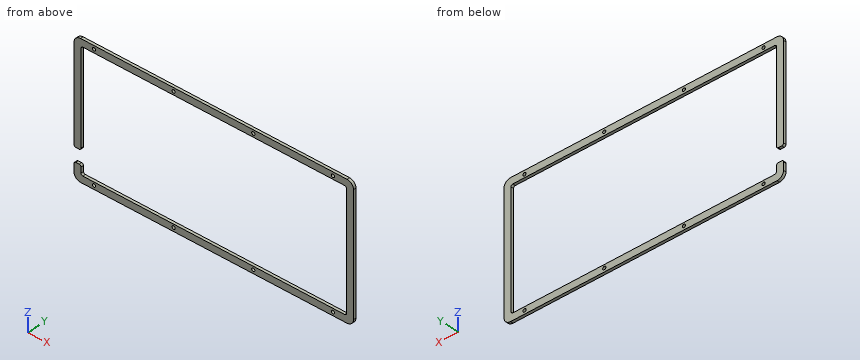
from build123d import *

# Parameters (mm, degrees)
SKETCH1_W           = 350
SKETCH1_H           = 200
BOSS_EXTRUDE1_DEPTH = 3
SKETCH2_OUTSIDE_W   = 432.624
SKETCH2_OUTSIDE_H   = 282.624
SKETCH2_OUTSIDE_R   = 1.7
CUT_EXTRUDE1_DEPTH  = 10


with BuildPart() as part:
    # Sketch1 → Boss-Extrude1 (new body)
    with BuildSketch(Plane(origin=(0, 0, 0), x_dir=(1, 0, 0), z_dir=(0, 1, 0))):
        with Locations((175, 100)):
            Rectangle(SKETCH1_W, SKETCH1_H)
    extrude(amount=BOSS_EXTRUDE1_DEPTH)

    # Sketch2 outside → Cut-Extrude1 (cut)
    with BuildSketch(Plane(origin=(0, 3, 0), x_dir=(1, 0, 0), z_dir=(0, 1, 0))):
        with Locations((175, 100)):
            Rectangle(SKETCH2_OUTSIDE_W, SKETCH2_OUTSIDE_H)
        with BuildLine():
            Line((334.453835379, 22.4974157), (46.754485379, 22.4974157))
            ThreePointArc((46.754485379, 22.4974157), (41.80473791, 24.547668232), (39.754485379, 29.4974157))
            Line((39.754485379, 29.4974157), (39.754485379, 132.1968757))
            ThreePointArc((39.754485379, 132.1968757), (40.340271816, 133.611089262), (41.754485379, 134.1968757))
            Line((41.754485379, 134.1968757), (45.254485379, 134.1968757))
            ThreePointArc((45.254485379, 134.1968757), (46.668698941, 133.611089262), (47.254485379, 132.1968757))
            Line((47.254485379, 132.1968757), (47.254485379, 31.9974157))
            ThreePointArc((47.254485379, 31.9974157), (47.840271816, 30.583202138), (49.254485379, 29.9974157))
            Line((49.254485379, 29.9974157), (331.953835379, 29.9974157))
            ThreePointArc((331.953835379, 29.9974157), (333.368048941, 30.583202138), (333.953835379, 31.9974157))
            Line((333.953835379, 31.9974157), (333.953835379, 157.1968757))
            ThreePointArc((333.953835379, 157.1968757), (333.368048941, 158.611089262), (331.953835379, 159.1968757))
            Line((331.953835379, 159.1968757), (49.254485379, 159.1968757))
            ThreePointArc((49.254485379, 159.1968757), (47.840271816, 158.611089262), (47.254485379, 157.1968757))
            Line((47.254485379, 157.1968757), (47.254485379, 151.1968757))
            ThreePointArc((47.254485379, 151.1968757), (46.668698941, 149.782662138), (45.254485379, 149.1968757))
            Line((45.254485379, 149.1968757), (41.754485379, 149.1968757))
            ThreePointArc((41.754485379, 149.1968757), (40.340271816, 149.782662138), (39.754485379, 151.1968757))
            Line((39.754485379, 151.1968757), (39.754485379, 159.6968757))
            ThreePointArc((39.754485379, 159.6968757), (41.80473791, 164.646623168), (46.754485379, 166.6968757))
            Line((46.754485379, 166.6968757), (334.453835379, 166.6968757))
            ThreePointArc((334.453835379, 166.6968757), (339.403582847, 164.646623168), (341.453835379, 159.6968757))
            Line((341.453835379, 159.6968757), (341.453835379, 29.4974157))
            ThreePointArc((341.453835379, 29.4974157), (339.403582847, 24.547668232), (334.453835379, 22.4974157))
        make_face(mode=Mode.SUBTRACT)
        with Locations((319.254485379, 26.4974157)):
            Circle(SKETCH2_OUTSIDE_R)
        with Locations((233.254485379, 26.2474157)):
            Circle(SKETCH2_OUTSIDE_R)
        with Locations((61.254485379, 26.2474157)):
            Circle(SKETCH2_OUTSIDE_R)
        with Locations((147.254485379, 26.2474157)):
            Circle(SKETCH2_OUTSIDE_R)
        with Locations((319.254485379, 162.9468757)):
            Circle(SKETCH2_OUTSIDE_R)
        with Locations((233.254485379, 162.6968757)):
            Circle(SKETCH2_OUTSIDE_R)
        with Locations((61.254485379, 162.6968757)):
            Circle(SKETCH2_OUTSIDE_R)
        with Locations((147.254485379, 162.6968757)):
            Circle(SKETCH2_OUTSIDE_R)
    extrude(amount=-CUT_EXTRUDE1_DEPTH, mode=Mode.SUBTRACT)


solid = part.part
Source: CAD feature listing. Evaluate the final solid. Frame: model axes, mm. Give positions to 0.01 mm unless a question says otherwise; leave off trailing zeros. Write each loop counter-clockwise with the first axis right and the second up, starting at its lowest first coordinate (ties: lowest second). Pieces come first, ordered by that corner, then holes. Notation, with made-up numbers: (56.5, 59.5) -> (109.5, 59.5) arc R24 ccw to (109.5, 81.5) -> close; hole circle Ø9 at (47, 4.25). An arc over 180 degrees is marked (long way). Write item = value, one per line.
Q1. Cut plane C-C on y = 1.95. State how many separate pieces and enclosed holes the cut face has, then the cut area to 3 significant figures.
Here are the results:
separate_pieces = 1
enclosed_holes = 8
area = 6,240 mm²
Q2. Cut plane D-D on z = -137. Return loops of the section in (x, y).
Here are the results:
outline = (333.95, 0) -> (341.45, 0) -> (341.45, 3) -> (333.95, 3) -> close
Q3. First-contact query: pin 1 (2.5 mm diameter, centred on x = 147.25, z = -162.7, fed in from -Y); pin 2 (5.5 mm diameter, centred on x = 233.25, z = -26.25, fed in from +Y); pin 3 (1.5 mm diameter, centred on x = 44.5, y = 1, fed in from +Z). Flat tips, straight axial feed; report the tip coordinate or a pass-through.
Here are the results:
pin_1 = through
pin_2 = 3
pin_3 = -22.66
Q4. Cut plane B-B on x = 197.5. Return loops of the section in (y, z).
Here are the results:
outline = (0, -166.7) -> (3, -166.7) -> (3, -159.2) -> (0, -159.2) -> close; (0, -30) -> (3, -30) -> (3, -22.5) -> (0, -22.5) -> close
Q5. Cut plane A-A on z = -63. Return loops of the section in (x, y), then the cut area to 3 significant figures.
Here are the results:
outline = (39.75, 0) -> (47.25, 0) -> (47.25, 3) -> (39.75, 3) -> close; (333.95, 0) -> (341.45, 0) -> (341.45, 3) -> (333.95, 3) -> close
area = 45.0 mm²
Q6. Line query: line 1 (Z direction, x = 303, y = 0.1); line 2 (X direction, y = 2.8, z = -156); line 3 (X direction, y = 2.45, z = -141). Output: solid intervals per line, ascending. Write a range as from..to.
Here are the results:
line_1 = -166.7..-159.2, -30..-22.5
line_2 = 39.75..47.25, 333.95..341.45
line_3 = 333.95..341.45
